Source: CAD feature listing. Evaluate the final solid. Frame: model axes, mm. Face numbers are marked on the shaded views. A direction names the side the tool comes from. Round coordinates to 2 decimals unless told otherwise and drop trailing zeros. Loops run counter-clockwise (first coordinate to the right, second up) from the corner with the lowest first, then second, coordinate; pieces in that order, holes last. Notation, with made-up numbers: (-24.75, -14.5) - (-7.75, -14.5) arc R18 ccw to (-7.75, 13.5) - close; hole circle Ø11 at (87.25, 18). An arc over 180 degrees is marked (long way). One line per question, with ' | ' between items.
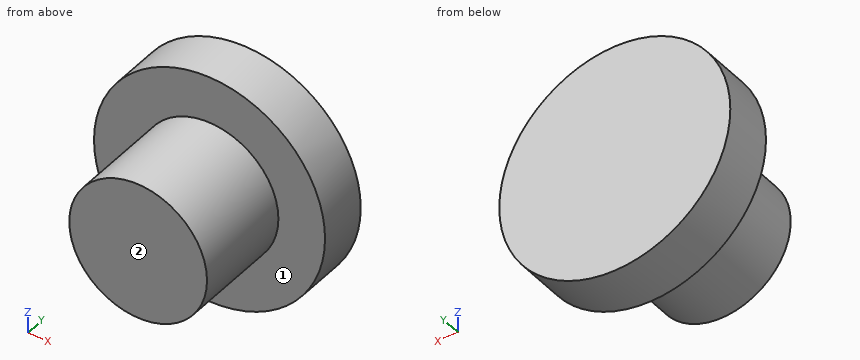
from build123d import *

# Parameters (mm, degrees)
F0_R     = 11.566794
F1_DEPTH = 5.08
F2_R     = 6.495217
F3_DEPTH = 2.54
F4_R     = 6.897415
F5_DEPTH = 12.7


with BuildPart() as f1:
    # F0 (on Front) → F1 (new body)
    with BuildSketch(Plane.XZ):
        with Locations((-44.537589, 34.487069)):
            Circle(F0_R)
    extrude(amount=F1_DEPTH)

    # F2 (on face) → F3 (cut)
    with BuildSketch(Plane.XZ.offset(5.08)):
        with Locations((-44.537589, 34.487069)):
            Circle(F2_R)
    extrude(amount=-F3_DEPTH, mode=Mode.SUBTRACT)

    # F4 (on face) → F5 (join)
    with BuildSketch(Plane.XZ.offset(2.54)):
        with Locations((-44.537589, 34.487069)):
            Circle(F4_R)
    extrude(amount=F5_DEPTH)


solid = f1.part
1. Access query for the marked faces 1 and 2. Directions: +Z, -Z, +X, -X, +Y, -Y. A direction counts if a zero-diameter tool reaches every point of the face in a straight line with its end or side. Return the directions, or none.
Worked out:
face 1: -Y | face 2: +Z, -Z, +X, -X, -Y
2. Section query A-A, the plane z = 28.5. Return loops of the section in (x, y).
Worked out:
outline: (-54.43, -5.08) - (-47.96, -5.08) - (-47.96, -15.24) - (-41.11, -15.24) - (-41.11, -5.08) - (-34.64, -5.08) - (-34.64, 0) - (-54.43, 0) - close
3. Section query D-D, the plane x = -36.25. Return loops of the section in (y, z), plus the area to 3 significant figures.
Worked out:
outline: (-5.08, 26.42) - (0, 26.42) - (0, 42.56) - (-5.08, 42.56) - close | area: 82.0 mm2
4. Contact query for flat-ended pins moving along their axis: P1, Ø4, axis at y = -4.5, z = 38.5, coming from the -X side; P2, Ø6, axis at x = -41.5, y = -9.5, coming from the -Z side; P3, Ø5, axis at x = -46.5, z = 26, coming from the -Y side; P4, Ø1.5, axis at y = -1.5, z = 31, coming from the -X side. Output: stop coordinate, or through.
Worked out:
P1: stops at x = -55.93 | P2: stops at z = 27.59 | P3: stops at y = -15.24 | P4: stops at x = -55.78
5. Material intervals for probe 1 along Y at (x, z) = (-35.75, 28.5); probe 2 along Z at (x, y) = (-40.25, -9); probe 3 along Z at (x, y) = (-49.75, -1.75), sorted ascending.
Worked out:
probe 1: y = -5.08 to 0 | probe 2: z = 29.08 to 39.89 | probe 3: z = 24.16 to 44.81
6. Section query B-B, the plane x = -50. Return loops of the section in (y, z).
Worked out:
outline: (-15.24, 30.28) - (-5.08, 30.28) - (-5.08, 24.29) - (0, 24.29) - (0, 44.68) - (-5.08, 44.68) - (-5.08, 38.7) - (-15.24, 38.7) - close
7. Section query C-C, the plane y = -1.5. Return loops of the section in (x, z), plus the area to 3 significant figures.
Worked out:
outline: circle Ø23.13 at (-44.54, 34.49) | area: 420 mm2
